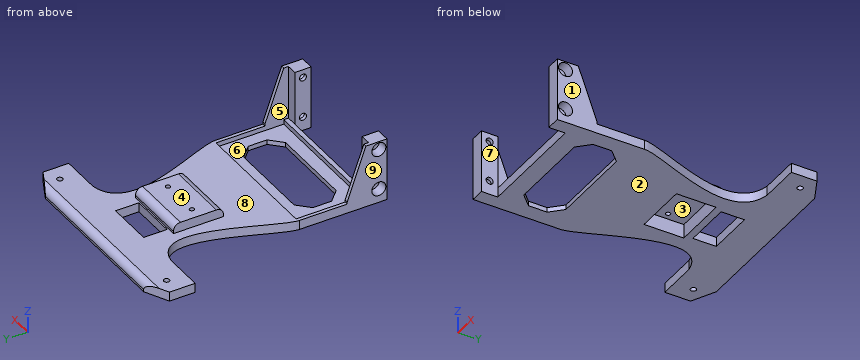
```python
from build123d import *

# Parameters (mm, degrees)
F0_W      = 46
F0_H      = 18
F0_R      = 1.2
F0_W_2    = 23
F0_H_2    = 17
F0_W_3    = 20
F0_H_3    = 10
F1_DEPTH  = 4
F2_SIZE2  = 5
F2_SIZE   = 10
F3_SIZE2  = 10
F3_SIZE   = 5
F4_SIZE   = 5
F5_W      = 1.5
F5_H      = 10
F6_DEPTH  = 27
F7_R      = 1.5
F8_DEPTH  = 60
F9_R      = 3
F10_DEPTH = 4.5
F11_R     = 3
F12_DEPTH = 4.5
F13_W     = 57
F13_H     = 29
F14_DEPTH = 2
F15_SIZE2 = 22
F15_SIZE  = 8
F16_SIZE2 = 8
F16_SIZE  = 22
F17_W     = 27
F17_H     = 21.3817437291
F17_W_2   = 23
F17_H_2   = 17
F18_DEPTH = 2
F19_W     = 27
F19_H     = 21.3817437291
F20_DEPTH = 2
F21_R     = 1
F22_DEPTH = 2
F23_R     = 3


with BuildPart() as f1:
    # F0 (on Top) → F1 (new body)
    with BuildSketch(Plane.XY):
        with BuildLine():
            Line((0, 84), (-45, 84))
            Line((-45, 84), (-45, 68))
            Line((-45, 68), (-30, 68))
            Line((-30, 68), (-27.8254859149, 68))
            add(Edge.make_bspline(
                [(-27.8254859149, 68), (-4.1811005212, 64), (-30, 23.7322062403), (-30, 14.3733293898)],
                knots=[0, 0, 0, 0, 53.6707398145, 53.6707398145, 53.6707398145, 53.6707398145], degree=3))
            Line((-30, 14.3733293898), (-30, -16))
            Line((-30, -16), (0, -16))
            Line((0, -16), (30, -16))
            Line((30, -16), (30, 14.3733293898))
            add(Edge.make_bspline(
                [(27.8254859149, 68), (4.1811005212, 64), (30, 23.7322062403), (30, 14.3733293898)],
                knots=[0, 0, 0, 0, 53.6707398145, 53.6707398145, 53.6707398145, 53.6707398145], degree=3))
            Line((27.8254859149, 68), (30, 68))
            Line((30, 68), (45, 68))
            Line((45, 68), (45, 84))
            Line((45, 84), (0, 84))
        make_face()
        with Locations((0, 0.500412114)):
            Rectangle(F0_W, F0_H, mode=Mode.SUBTRACT)
        with Locations((-38, 76)):
            Circle(F0_R, mode=Mode.SUBTRACT)
        with Locations((0, 47.5)):
            Rectangle(F0_W_2, F0_H_2, mode=Mode.SUBTRACT)
        with Locations((0, 64)):
            Rectangle(F0_W_3, F0_H_3, mode=Mode.SUBTRACT)
        with Locations((38, 76)):
            Circle(F0_R, mode=Mode.SUBTRACT)
    extrude(amount=F1_DEPTH)

    # F2
    f2_edges = [f1.edges().sort_by_distance(p)[0] for p in [
        (45, 84, 2),
    ]]
    f2_side = f1.faces().sort_by_distance((0, 84, 2))[0]
    chamfer(f2_edges, length=F2_SIZE, length2=F2_SIZE2, reference=f2_side)

    # F3
    f3_edges = [f1.edges().sort_by_distance(p)[0] for p in [
        (-45, 84, 2),
    ]]
    f3_side = f1.faces().sort_by_distance((-45, 76, 2))[0]
    chamfer(f3_edges, length=F3_SIZE, length2=F3_SIZE2, reference=f3_side)

    # F4
    f4_edges = [f1.edges().sort_by_distance(p)[0] for p in [
        (-23, 9.500412, 2),
        (23, 9.500412, 2),
        (23, -8.499588, 2),
        (-23, -8.499588, 2),
    ]]
    chamfer(f4_edges, length=F4_SIZE)

    # F5 (on Top) → F6 (join)
    with BuildSketch(Plane.XY):
        Polygon((-24, -16), (-28.5, -16), (-28.5, -6), (-30, -6), (-30, -16), (-30, -23), (-24, -23), align=None)
        Polygon((30, -23), (30, -16), (28.5, -16), (24, -16), (24, -23), align=None)
        with Locations((29.25, -11)):
            Rectangle(F5_W, F5_H)
    extrude(amount=F6_DEPTH)

    # F7 (on face) → F8 (cut)
    with BuildSketch(Plane.YZ.offset(30)):
        with Locations((-19.5, 23.5)):
            Circle(F7_R)
        with Locations((-19.5, 6)):
            Circle(F7_R)
    extrude(amount=-F8_DEPTH, mode=Mode.SUBTRACT)

    # F9 (on face) → F10 (cut)
    with BuildSketch(Plane.YZ.offset(30)):
        with Locations((-19.5, 23.5)):
            Circle(F9_R)
        with Locations((-19.5, 6)):
            Circle(F9_R)
    extrude(amount=-F10_DEPTH, mode=Mode.SUBTRACT)

    # F11 (on face) → F12 (cut)
    with BuildSketch(Plane(origin=(-30, 0, 0), x_dir=(0, -1, 0), z_dir=(-1, 0, 0))):
        with Locations((19.5, 23.5)):
            Circle(F11_R)
        with Locations((19.5, 6)):
            Circle(F11_R)
    extrude(amount=-F12_DEPTH, mode=Mode.SUBTRACT)

    # F13 (on face) → F14 (cut)
    with BuildSketch(Plane.XY.offset(4)):
        with Locations((0, 0.5)):
            Rectangle(F13_W, F13_H)
    extrude(amount=-F14_DEPTH, mode=Mode.SUBTRACT)

    # F15
    f15_edges = [f1.edges().sort_by_distance(p)[0] for p in [
        (29.25, -6, 27),
    ]]
    f15_side = f1.faces().sort_by_distance((27.592105, -17.263158, 27))[0]
    chamfer(f15_edges, length=F15_SIZE, length2=F15_SIZE2, reference=f15_side)

    # F16
    f16_edges = [f1.edges().sort_by_distance(p)[0] for p in [
        (-29.25, -6, 27),
    ]]
    f16_side = f1.faces().sort_by_distance((-29.25, -6, 15.5))[0]
    chamfer(f16_edges, length=F16_SIZE, length2=F16_SIZE2, reference=f16_side)

    # F17 (on face) → F18 (join)
    with BuildSketch(Plane.XY.offset(4)):
        with Locations((0, 47.6908718646)):
            Rectangle(F17_W, F17_H)
        with Locations((0, 47.5)):
            Rectangle(F17_W_2, F17_H_2, mode=Mode.SUBTRACT)
    extrude(amount=F18_DEPTH)

    # F19 (on face) → F20 (join)
    with BuildSketch(Plane.XY.offset(6)):
        with Locations((0, 47.6908718646)):
            Rectangle(F19_W, F19_H)
    extrude(amount=F20_DEPTH)

    # F21 (on face) → F22 (cut)
    with BuildSketch(Plane.XY.offset(8)):
        with Locations((-8.5, 47.5)):
            Circle(F21_R)
        with Locations((8.5, 47.5)):
            Circle(F21_R)
    extrude(amount=-F22_DEPTH, mode=Mode.SUBTRACT)

    # F23
    f23_edges = [f1.edges().sort_by_distance(p)[0] for p in [
        (0, 58.381744, 8),
        (0, 84, 4),
        (0, 37, 8),
    ]]
    fillet(f23_edges, radius=F23_R)


solid = f1.part
```
Could you check a few things on this model? Use its own coordinates, in mm. Face numbers are marked on the shaded views. A direction names the side the tool comes from. Give positions to 0.01 mm unless a question says otherwise; leave off trailing zeros. Order: outer loops, then holes, each group sorted by start corner. A loop starts at its lowest first (then second) coordinate and runs counter-clockwise, first axis right, second up.
Q1. If I drill on line 1 along Z through (x, y) = (-24.5, -19.5); line 2 along X through (y, z) = (-14.5, 4.75); line 3 along Z through (x, y) = (-28, -19), over which ranges is the centre line in solid material (lowest first)?
Q2. I'm going to push flat-ended pins straight in: P1, Ø1.5, axis at x = 0.5, y = 33, coming from the +Z side; P2, Ø3.5, axis at y = -19.5, z = 23.5, coming from the +X side; P3, Ø1.6, axis at x = -1, z = 3.5, coming from the -Y side. Where does each tip first touch, or does it pass through?
Q3. Suppose I cut it at B-B, the plane x = 2. Write out the boundary of the cut face in (y, z), and give its area (3 significant figures).
Q4. Suppose I cut it at D-D, the plane x = -38. Write out the boundary of the cut face in (y, z), and give its area (3 significant figures).
Q5. We'd pull the mould along X, two halves only. Please class the marked faces 6, 7, 8 and 9: +X half, -X half, draft (parallel to the pull), parting line (faces both ways), or undercut.
Q6. Suppose I cut it at A-A, the plane y = 76. Write out the boundary of the cut face in (x, z), and give its area (3 significant figures).
Q7. For the marked faces 1, 2, 3, 4 and 5, which set-ups out of +Z, -Z, +X, -X, +Y, -Y let a thin tool reach every point of the face, with its end or its side?
Q8. Suppose I cut it at C-C, the plane z = 10.5. Write out the boundary of the cut face in (x, y).
Solution:
1. line 1: z = 0 to 4.5, 7.5 to 22, 25 to 27
1. line 2: x = -30 to -28.5, 28.5 to 30
1. line 3: z = 0 to 3.04, 8.96 to 20.54, 26.46 to 27
2. P1: stops at z = 4
2. P2: stops at x = 25.5
2. P3: stops at y = -16
3. outline: (-16, 0) - (-8.5, 0) - (-8.5, 2) - (-14, 2) - (-14, 4) - (-16, 4) - close; (9.5, 0) - (39, 0) - (39, 6) - (56, 6) - (56, 0) - (59, 0) - (59, 4) - (58.38, 4) - (58.38, 5) arc R3 ccw to (55.38, 8) - (40, 8) arc R3 ccw to (37, 5) - (37, 4) - (15, 4) - (15, 2) - (9.5, 2) - close; (69, 0) - (84, 0) - (84, 1) arc R3 ccw to (81, 4) - (69, 4) - close
3. area: 244 mm2
4. outline: (68, 0) - (74.8, 0) - (74.8, 4) - (68, 4) - close; (77.2, 0) - (82.5, 0) - (82.5, 3.6) arc R3 ccw to (81, 4) - (77.2, 4) - close
4. area: 48.2 mm2
5. face 6: undercut
5. face 7: undercut
5. face 8: draft
5. face 9: -X half
6. outline: (-45, 0) - (-39.2, 0) - (-39.2, 4) - (-45, 4) - close; (-36.8, 0) - (36.8, 0) - (36.8, 4) - (-36.8, 4) - close; (39.2, 0) - (45, 0) - (45, 4) - (39.2, 4) - close
6. area: 341 mm2
7. face 1: +Z, -Z, +X, -Y
7. face 2: -Z, +X, -X, +Y, -Y
7. face 3: -Z
7. face 4: +Z, +X, -X, +Y, -Y
7. face 5: +Z
8. outline: (-30, -23) - (-24, -23) - (-24, -16) - (-28.5, -16) - (-28.5, -8) - (-30, -8) - close; (24, -23) - (30, -23) - (30, -8) - (28.5, -8) - (28.5, -16) - (24, -16) - close
